For this review, take the finished solid that the model builds, in its own axes (mm). Face numbers are marked on the shaded views. A direction names the side the tool comes from. Give positions to 0.01 mm unless a question says otherwise; leave off trailing zeros. Write each loop counter-clockwise with the first axis right and the second up, starting at its lowest first coordinate (ties: lowest second). Pieces come first, ordered by that corner, then holes. Notation, with made-up numbers: (-32, 3) -> (-20, 3) arc R20 cw to (-20, 38) -> close; hole circle Ø9 at (25, -40). An arc over 180 degrees is marked (long way). Write item = value, one per line.
```python
from build123d import *

# Parameters (mm, degrees)
F0_W     = 101.6
F0_H     = 50.8
F0_R     = 1.65
F1_DEPTH = 1.6
F2_W     = 15.501738
F2_H     = 12.617692
F2_W_2   = 33.887516
F2_H_2   = 15.411611
F2_W_3   = 41.007504
F2_H_3   = 23.252605
F2_W_4   = 16.853633
F2_H_4   = 22.441468
F2_R     = 4.087607
F2_R_2   = 3.08016
F2_R_3   = 2.845767
F3_DEPTH = 27


with BuildPart() as f1:
    # F0 (on Top) → F1 (new body)
    with BuildSketch(Plane.XY):
        with Locations((-19.175592, 1.734423)):
            Rectangle(F0_W, F0_H)
        with Locations((-66.800592, -20.890577)):
            Circle(F0_R, mode=Mode.SUBTRACT)
        with Locations((28.449408, -20.890577)):
            Circle(F0_R, mode=Mode.SUBTRACT)
        with Locations((-66.800592, 23.559423)):
            Circle(F0_R, mode=Mode.SUBTRACT)
        with Locations((28.449408, 23.559423)):
            Circle(F0_R, mode=Mode.SUBTRACT)
    extrude(amount=F1_DEPTH)

    # F2 (on face) → F3 (join)
    with BuildSketch(Plane.XY.offset(1.6)):
        with Locations((-50.060928, 15.461646)):
            Rectangle(F2_W, F2_H)
        with Locations((-20.229096, 14.154814)):
            Rectangle(F2_W_2, F2_H_2)
        with Locations((-28.295409, -10.224371)):
            Rectangle(F2_W_3, F2_H_3)
        with Locations((2.708067, -6.484127)):
            Rectangle(F2_W_4, F2_H_4)
        with Locations((15.460948, 17.714806)):
            Circle(F2_R)
        with Locations((14.379433, 7.620651)):
            Circle(F2_R_2)
        with Locations((15.280697, -3.28464)):
            Circle(F2_R_3)
    extrude(amount=F3_DEPTH)


solid = f1.part
```
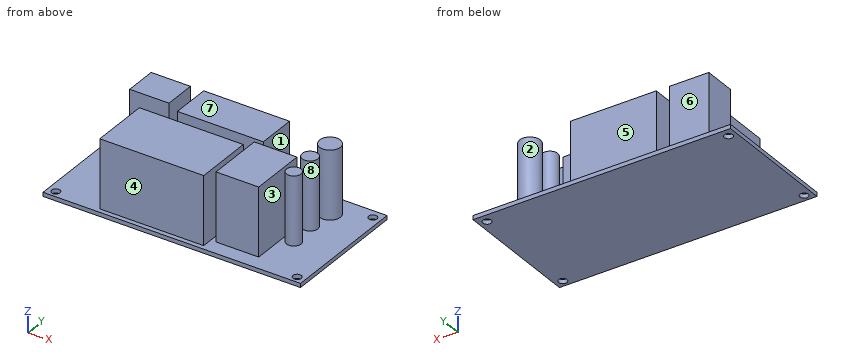
(1) Take a section at B-B (z = 16.5). Write out the cut boundary in (x, y).
Answers below:
outline = (-57.81, 9.15) -> (-42.31, 9.15) -> (-42.31, 21.77) -> (-57.81, 21.77) -> close; (-48.8, -21.85) -> (-7.79, -21.85) -> (-7.79, 1.4) -> (-48.8, 1.4) -> close; (-37.17, 6.45) -> (-3.29, 6.45) -> (-3.29, 21.86) -> (-37.17, 21.86) -> close; (-5.72, -17.7) -> (11.13, -17.7) -> (11.13, 4.74) -> (-5.72, 4.74) -> close; circle Ø6.16 at (14.38, 7.62); circle Ø8.18 at (15.46, 17.71); circle Ø5.69 at (15.28, -3.28)
(2) For pin 1 (7.5 mm diameter, centred on y = 12, z = 17.5, fed in from -X); pin 2 (2 mm diameter, centred on x = -38, z = 3, fed in from +Y); pin 3 (8.5 mm diameter, centred on x = -1, z = 16, fed in from -Y); pin 4 (3 mm diameter, centred on x = -66.8, y = 23.56, fed in from -Z), all flat-tipped, find the tip position at first contact; note any pin that passes through.
Answers below:
pin_1 = -57.81
pin_2 = 21.86
pin_3 = -17.7
pin_4 = through
(3) Tool access review of the marked faces 1, 2, 3, 4 and 5: name each direction out of +Z, -Z, +X, -X, +Y, -Y from which nothing blocks a thin tool from reaching the whole face with its end or side.
Answers below:
face_1 = +Z, +Y
face_2 = +Z
face_3 = +Z, +Y, -Y
face_4 = +Z, +X, -X, -Y
face_5 = +Z, +X, -X, +Y
(4) Take a section at D-D (x = -54). Write out the cut boundary in (y, z).
Answers below:
outline = (-23.67, 0) -> (27.13, 0) -> (27.13, 1.6) -> (21.77, 1.6) -> (21.77, 28.6) -> (9.15, 28.6) -> (9.15, 1.6) -> (-23.67, 1.6) -> close
(5) Take a section at A-A (x = -32). Write out the cut boundary in (y, z), plus the area to 3 significant figures.
Answers below:
outline = (-23.67, 0) -> (27.13, 0) -> (27.13, 1.6) -> (21.86, 1.6) -> (21.86, 28.6) -> (6.45, 28.6) -> (6.45, 1.6) -> (1.4, 1.6) -> (1.4, 28.6) -> (-21.85, 28.6) -> (-21.85, 1.6) -> (-23.67, 1.6) -> close
area = 1,130 mm^2
(6) The part is to be moulded in two halves that separate along Y. For the marked faces 6, 7 and 8, say which applies: released by +Y, released by -Y, zero draft, split by the parting line, or undercut.
Answers below:
face_6 = released by +Y
face_7 = zero draft
face_8 = undercut
(7) Take a section at C-C (y = -16). Write out the cut boundary in (x, z).
Answers below:
outline = (-69.98, 0) -> (31.62, 0) -> (31.62, 1.6) -> (11.13, 1.6) -> (11.13, 28.6) -> (-5.72, 28.6) -> (-5.72, 1.6) -> (-7.79, 1.6) -> (-7.79, 28.6) -> (-48.8, 28.6) -> (-48.8, 1.6) -> (-69.98, 1.6) -> close
(8) To check wall thickness, follow probe 1 along Y at (x, z) = (-29.5, 12); probe 2 along Y at (x, z) = (-48.5, 17); probe 3 along X at (y, z) = (-9, 7.75). State the ranges of each line that lie inside material, in increasing order.
Answers below:
probe_1 = -21.85 to 1.4, 6.45 to 21.86
probe_2 = -21.85 to 1.4, 9.15 to 21.77
probe_3 = -48.8 to -7.79, -5.72 to 11.13
